The figure shows three views and two pictorial views of one solid part (mm, origin at its lowest corner). Answer the questions. A direction names the side the tool comes from. Round coordinates to 2 decimals unless told otherwise and drop trailing zeros. Order: outer loops, then holes, each group sorted by start corner. A loop starts at its lowest first (then second) coordinate and runs counter-clockwise, first axis right, second up. Notation, with made-up numbers: (31, -5) -> (39, -5) arc R33 cw to (39, 32) -> close; hole circle Ø3 at (78.25, -14.75). An arc over 180 degrees is marked (long way). One line per item, written item: value. Start each with the question number.
1. Section A-A (y = 9.75) is taken. Give the vertices of the cut face in (x, z), then the cut area to 3 significant figures.
2. Consider line 1 (X direction, y = 20.75, z = 28.5); line 2 (Z direction, x = 156.5, y = 24.5). Determine where each line is inside the solid, lowest interval first.
3. For the marked faces 1, 2 and 3, determine the directions among +Z, -Z, +X, -X, +Y, -Y from which every point of the face is accessible in a straight line to the end or side of a thin tool.
4. Flat-ended cylindrical pins translate along their axes: pin 1 Ø8 at (x, y) = (3.5, 10) entering from -Z; pin 2 Ø3 at (x, y) = (3, 20) entering from +Z; pin 3 Ø3 at (x, z) = (6.5, 16) entering from +Y. Find the tip coordinate at first contact, or state that the pin passes through.
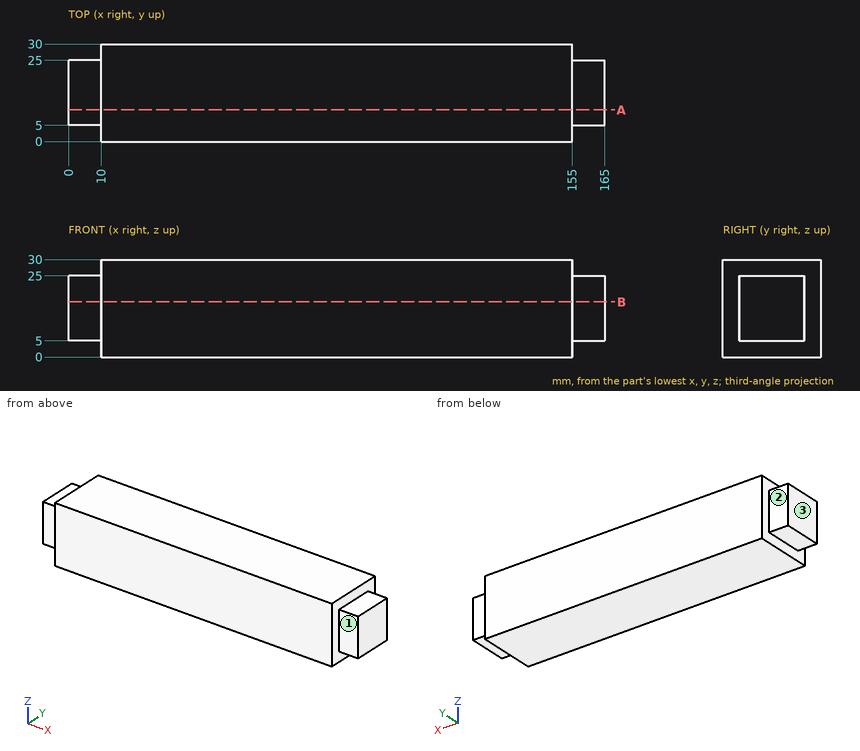
Answer:
1. outline: (0, 5) -> (10, 5) -> (10, 0) -> (155, 0) -> (155, 5) -> (165, 5) -> (165, 25) -> (155, 25) -> (155, 30) -> (10, 30) -> (10, 25) -> (0, 25) -> close
1. area: 4,750 mm^2
2. line 1: 10 to 155
2. line 2: 5 to 25
3. face 1: +Z, -Z, +X, -Y
3. face 2: +Z, -Z, -X, +Y
3. face 3: +Z, -Z, -X, +Y, -Y
4. pin 1: z = 5
4. pin 2: z = 25
4. pin 3: y = 25
